Autodesk Inventor part; units mm, degrees
ref_plane "YZ Plane" through (0, 0, 0) normal (1, 0, 0) x (0, 1, 0)
ref_plane "XZ Plane" through (0, 0, 0) normal (0, 1, 0) x (-1, 0, 0)
ref_plane "XY Plane" through (0, 0, 0) normal (0, 0, 1) x (1, 0, 0)
sketch "Sketch1" plane through (0, 0, 0) normal (0, 1, 0) x (-1, 0, 0)
  line L0 (0, 0) -> (0, 38.1)
  line L1 (0, 38.1) -> (88.9, 38.1)
  line L2 (88.9, 38.1) -> (88.9, 0)
  line L3 (88.9, 0) -> (0, 0)
  circle A0 centre (19.8437, 12.7) radius 2.54
  circle A1 centre (19.8437, 25.4) radius 2.54
  circle A2 centre (69.0563, 25.4) radius 2.54
  circle A3 centre (69.0563, 12.7) radius 2.54
  circle A4 centre (6.35, 31.75) radius 3.302
  circle A5 centre (6.35, 6.35) radius 3.302
  circle A6 centre (82.55, 31.75) radius 3.302
  circle A7 centre (82.55, 6.35) radius 3.302
  line L4 (63.5, 28.575) -> (63.5, 9.525)
  line L5 (63.5, 9.525) -> (25.4, 9.525)
  line L6 (25.4, 9.525) -> (25.4, 28.575)
  line L7 (25.4, 28.575) -> (63.5, 28.575)
  dimension "d0" = 38.1
  dimension "d1" = 88.9
  dimension "d2" = 5.08
  dimension "d3" = 5.08
  dimension "d4" = 5.08
  dimension "d5" = 5.08
  dimension "d6" = 12.7
  dimension "d7" = 12.7
  dimension "d8" = 12.7
  dimension "d9" = 12.7
  dimension "d10" = 49.2125
  dimension "d11" = 49.2125
  dimension "d12" = 19.8438
  dimension "d14" = 19.8438
  dimension "d15" = 6.604
  dimension "d16" = 6.604
  dimension "d17" = 6.604
  dimension "d18" = 6.604
  dimension "d19" = 25.4
  dimension "d20" = 6.35
  dimension "d21" = 6.35
  dimension "d22" = 6.35
  dimension "d23" = 6.35
  dimension "d24" = 6.35
  dimension "d25" = 25.4
  dimension "d26" = 6.35
  dimension "d27" = 19.05
  dimension "d28" = 38.1
  dimension "d29" = 9.525
  dimension "d30" = 25.4
  dimension "d33" = 6.35
  dimension "d34" = 76.2
extrude "Extrusion1" add sketch "Sketch1" along normal blind 25.4
properties part number "MotorHolder"
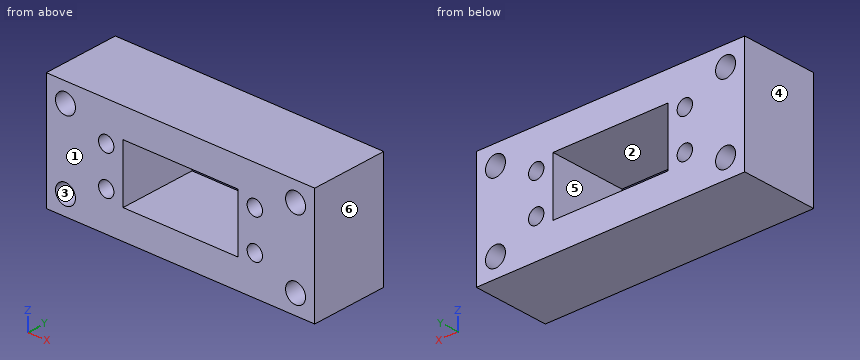
Model file for the job. Use its own axes, mm. Face numbers are marked on the shaded views. A direction names the side the tool comes from. Coordinates: 2 decimals unless noted, no trailing zeros. Order: outer loops, then holes, each group sorted by start corner. A loop starts at its lowest first (then second) coordinate and runs counter-clockwise, first axis right, second up. Notation, with made-up numbers: M 65,43.5 L 114,43.5 A29 ccw 114,68.5 Z; hole C -6,74 d4. An arc over 180 degrees is marked long. Return JSON: item names as keys, results as strings.
1. Tool access for the marked faces 5 and 6: list every direction of +Z, -Z, +X, -X, +Y, -Y with a clear straight run to the whole face (end or side of a thin tool).
Ans:
{"face 5": "+Y, -Y", "face 6": "+Z, -Z, +X, +Y, -Y"}
2. Saw through at D-D (x = -46). Give the cut face in (y, z) (3 decimals), and give its area (3 significant figures).
Ans:
{"outline": "M 0,0 L 25.4,0 L 25.4,9.525 L 0,9.525 Z; M 0,28.575 L 25.4,28.575 L 25.4,38.1 L 0,38.1 Z", "area": "484 mm^2"}
3. Saw through at A-A (x = -82.55). Give the cut face in (y, z).
Ans:
{"outline": "M 0,0 L 25.4,0 L 25.4,3.05 L 0,3.05 Z; M 0,9.65 L 25.4,9.65 L 25.4,28.45 L 0,28.45 Z; M 0,35.05 L 25.4,35.05 L 25.4,38.1 L 0,38.1 Z"}
4. Pull direction X, two halves, no side cores. Call the marked faces 1, 2, 3 and 4: +X half, -X half, draft (parallel to the pull), parting line (faces both ways), or undercut.
Ans:
{"face 1": "draft", "face 2": "undercut", "face 3": "undercut", "face 4": "-X half"}
5. Saw through at B-B (y = 12). Give the number of separate pieces and of enclosed holes in the cut face, and give its area (3 significant figures).
Ans:
{"separate pieces": "1", "enclosed holes": "9", "area": "2,440 mm^2"}
6. Saw through at C-C (z = 17). Give the cut face in (x, y).
Ans:
{"outline": "M -88.9,0 L -63.5,0 L -63.5,25.4 L -88.9,25.4 Z; M -25.4,0 L 0,0 L 0,25.4 L -25.4,25.4 Z"}
7. Drill centre lines: probe 1 along Z at (x, y) = (-82.55, 15); probe 2 along X at (y, z) = (4.5, 21); probe 3 along X at (y, z) = (11.75, 30). Where is each one in solid material? Low to high.
Ans:
{"probe 1": "0 to 3.05, 9.65 to 28.45, 35.05 to 38.1", "probe 2": "-88.9 to -63.5, -25.4 to 0", "probe 3": "-88.9 to -85.35, -79.75 to -9.15, -3.55 to 0"}
